Build history of the part. All positions in model axes, mm. Face numbers are marked on the shaded views. Round coordinates to 2 decimals unless told otherwise and drop trailing zeros. Loops run counter-clockwise (first coordinate to the right, second up) from the corner with the lowest first, then second, coordinate; pieces in that order, holes last. Notation, with made-up numbers: (-38, 48) - (16, 48) arc R15 cw to (16, 69) - close; hole circle Ø1 at (36.5, -32). An arc over 180 degrees is marked (long way). Put each result on its own line as item: value. Start each with the question number.
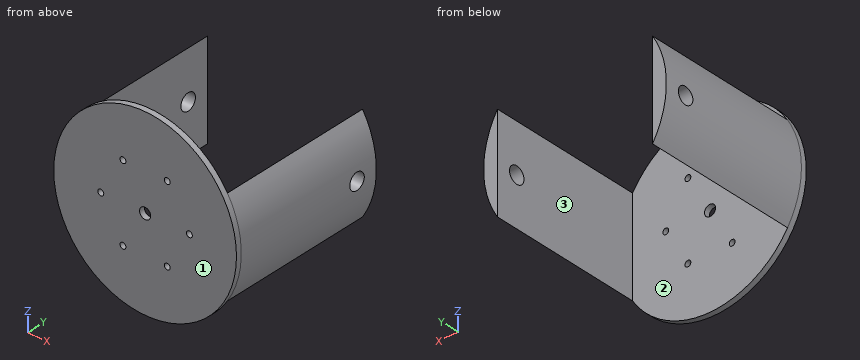
Autodesk Inventor part; units mm, degrees
ref_plane "Work Plane2" through (104.775, 0, 0) normal (1, 0, 0) x (0, 1, 0)
ref_plane "XZ Plane" through (0, 0, 0) normal (0, 1, 0) x (-1, 0, 0)
ref_plane "XY Plane" through (0, 0, 0) normal (0, 0, 1) x (1, 0, 0)
sketch "Sketch1" plane through (0, 0, 0) normal (0, 1, 0) x (-1, 0, 0)
  circle A0 centre (0, 0) radius 104.775
  dimension "baseOutsideDiameter" = 209.55
extrude "Extrusion1" add sketch "Sketch1" along normal blind 6.35
sketch "Sketch7" plane through (0, 6.35, 0) normal (0, 1, 0) x (1, 0, 0)
  line L0 (0, 0) -> (0, 104.775) construction
  circle A0 centre (0, 0) radius 104.775 construction
  line L1 (88.9, -55.449) -> (88.9, 55.449)
  arc A1 (88.9, -55.449) -> (88.9, 55.449) centre (0, 0) ccw
  dimension "spaceforTube" = 88.9
extrude "Extrusion7" add sketch "Sketch7" along normal blind 177.8
mirror "Mirror1" about plane through (0, 0, 0) normal (1, 0, 0) of "Extrusion7"
ref_plane "Work Plane2" through (104.775, 0, 0) normal (1, 0, 0) x (0, 1, 0)
sketch "Sketch8" plane through (104.775, 0, 0) normal (1, 0, 0) x (0, 1, 0)
  circle A0 centre (158.75, 0) radius 9.525
  line L0 (6.35, 55.449) -> (6.35, 104.775)
  point P0 (0, 0)
  dimension "d34" = 19.05
  dimension "holeHeight" = 152.4
extrude "Extrusion8" cut sketch "Sketch8" against normal through all
sketch "Sketch9" plane through (0, 0, 0) normal (0, -1, 0) x (1, 0, 0)
  circle A0 centre (0, 0) radius 6.35
  dimension "d47" = 12.7
extrude "Extrusion9" cut sketch "Sketch9" against normal through all
sketch "Sketch10" plane through (0, 0, 0) normal (0, -1, 0) x (1, 0, 0)
  point P0 (0, 0)
  point P1 (-50.8, 0)
  dimension "d50" = 50.8
hole "Hole1" at (-50.8, 0, 0) direction (0, 1, 0) diameter 6.7564 end through all
pattern_circular "Circular Pattern2" count 6 over 360 about axis through (0, -10, 0) along (0, 1, 0) of "Hole1"
equation "\"spaceforTube\" = bracketWidth + 0.5 * tubeDiameter"
equation "\"tubeDiameter\" = 165.1"
equation "\"bracketWidth\" = 6.35"
properties part number "topOfRaBase" material "ABS Plastic"
1) Slice it at B-B, the plane x = -2. Write the cut outline in (y, z).
2) Slice it at A-A, the plane y = 158.75. Write the cut outline in (x, z) (3 decimals), and give its area (3 significant figures).
3) Pull direction X, two halves, no side cores. Call the marked faces 1, 2 and 3: pulls with the +X half, pulls with the -X half, needs draft (parallel to the pull), parting line crosses it, or undercut.
4) Drill centre lines: line 1 (X direction, y = 34, z = -1); line 2 (Y direction, x = 96, z = 0) (3 decimals); line 3 (Y direction, x = 40.5, z = 96). Where is each one in solid material? Low to high. Write a range as [from, to].
5) Slice it at D-D, the plane z = -27.5. Write the cut outline in (x, y).
6) Drop flat-ended pins along their axis: pin 1 Ø9 at (x, z) = (-25.4, -43.99) entering from +Y; pin 2 Ø6 at (y, z) = (99.5, 17.5) entering from -X; pin 3 Ø11.5 at (x, z) = (0, 0) entering from +Y. Give the stop position or say it passes through.
7) Slice it at C-C, the plane y = 83. Write the cut outline in (x, z) (3 decimals).
Taken from the geometry:
1. outline: (0, -104.76) - (6.35, -104.76) - (6.35, -6.03) - (0, -6.03) - close; (0, 6.03) - (6.35, 6.03) - (6.35, 104.76) - (0, 104.76) - close
2. outline: (-104.341, -9.525) arc R104.775 ccw to (-88.9, -55.449) - (-88.9, -9.525) - close; (-104.341, 9.525) - (-88.9, 9.525) - (-88.9, 55.449) arc R104.775 ccw to start; (88.9, -55.449) arc R104.775 ccw to (104.341, -9.525) - (88.9, -9.525) - close; (88.9, 9.525) - (104.341, 9.525) arc R104.775 ccw to (88.9, 55.449) - close
2. area: 1,790 mm2
3. face 1: needs draft
3. face 2: undercut
3. face 3: undercut
4. line 1: x = [-104.77, -88.9], [88.9, 104.77]
4. line 2: y = [0, 149.225], [168.275, 184.15]
4. line 3: y = [0, 6.35]
5. outline: (-101.1, 0) - (101.1, 0) - (101.1, 184.15) - (88.9, 184.15) - (88.9, 6.35) - (-88.9, 6.35) - (-88.9, 184.15) - (-101.1, 184.15) - close
6. pin 1: stops at y = 6.35
6. pin 2: stops at x = -103.77
6. pin 3: passes through
7. outline: (-88.9, -55.449) - (-88.9, 55.449) arc R104.775 ccw to start; (88.9, -55.449) arc R104.775 ccw to (88.9, 55.449) - close
